from build123d import *

# Parameters (mm, degrees)
SKETCH_1_R          = 2.25
SKETCH_1_R_2        = 6
SKETCH_1_R_3        = 7.25
EXTRUDE_1_DEPTH     = 15
SKETCH_2_R          = 4.25
CUT_EXTRUDE_2_DEPTH = 8
SKETCH_3_R          = 3.4
CUT_EXTRUDE_3_DEPTH = 1188.655030604
SKETCH_4_R          = 5
CUT_EXTRUDE_4_DEPTH = 15


with BuildPart() as part:
    # 草图1 → 拉伸1 (new body)
    with BuildSketch(Plane.XY):
        with BuildLine():
            Line((1164.940753882, 1110.911631895), (1146.940753882, 1110.911631895))
            ThreePointArc((1146.940753882, 1110.911631895), (1143.405219976, 1109.4471658), (1141.940753882, 1105.911631895))
            Line((1141.940753882, 1105.911631895), (1141.940753882, 1045.911631895))
            Line((1141.940753882, 1045.911631895), (1145.440753882, 1045.911631895))
            Line((1145.440753882, 1045.911631895), (1145.440753882, 1020.911631895))
            ThreePointArc((1145.440753882, 1020.911631895), (1146.905219976, 1017.376097989), (1150.440753882, 1015.911631895))
            Line((1150.440753882, 1015.911631895), (1161.440753882, 1015.911631895))
            ThreePointArc((1161.440753882, 1015.911631895), (1164.976287788, 1017.376097989), (1166.440753882, 1020.911631895))
            Line((1166.440753882, 1020.911631895), (1166.440753882, 1045.911631895))
            Line((1166.440753882, 1045.911631895), (1185.940753882, 1045.911631895))
            Line((1185.940753882, 1045.911631895), (1185.940753882, 1060.411631895))
            Line((1185.940753882, 1060.411631895), (1165.827613848, 1060.411631895))
            ThreePointArc((1165.827613848, 1060.411631895), (1165.271903508, 1058.315850107), (1164.277525065, 1056.389110167))
            ThreePointArc((1164.277525065, 1056.389110167), (1164.426035256, 1053.42635052), (1161.46327561, 1053.574860711))
            ThreePointArc((1161.46327561, 1053.574860711), (1155.940753882, 1051.911631895), (1150.418232154, 1053.574860711))
            ThreePointArc((1150.418232154, 1053.574860711), (1147.455472508, 1053.42635052), (1147.603982698, 1056.389110167))
            ThreePointArc((1147.603982698, 1056.389110167), (1145.940753882, 1061.911631895), (1147.603982698, 1067.434153622))
            ThreePointArc((1147.603982698, 1067.434153622), (1147.455472508, 1070.396913269), (1150.418232154, 1070.248403078))
            ThreePointArc((1150.418232154, 1070.248403078), (1155.940753882, 1071.911631895), (1161.46327561, 1070.248403078))
            ThreePointArc((1161.46327561, 1070.248403078), (1164.426035256, 1070.396913269), (1164.277525065, 1067.434153622))
            ThreePointArc((1164.277525065, 1067.434153622), (1165.271903508, 1065.507413682), (1165.827613848, 1063.411631895))
            Line((1165.827613848, 1063.411631895), (1185.940753882, 1063.411631895))
            Line((1185.940753882, 1063.411631895), (1185.940753882, 1077.911631895))
            Line((1185.940753882, 1077.911631895), (1169.940753882, 1077.911631895))
            Line((1169.940753882, 1077.911631895), (1169.940753882, 1105.911631895))
            ThreePointArc((1169.940753882, 1105.911631895), (1168.476287788, 1109.4471658), (1164.940753882, 1110.911631895))
        make_face()
        with Locations((1162.940753882, 1104.911631895)):
            Circle(SKETCH_1_R, mode=Mode.SUBTRACT)
        with Locations((1155.940753882, 1097.911631895)):
            Circle(SKETCH_1_R_2, mode=Mode.SUBTRACT)
        with Locations((1148.940753882, 1104.911631895)):
            Circle(SKETCH_1_R, mode=Mode.SUBTRACT)
        with Locations((1148.940753882, 1090.911631895)):
            Circle(SKETCH_1_R, mode=Mode.SUBTRACT)
        with Locations((1162.940753882, 1090.911631895)):
            Circle(SKETCH_1_R, mode=Mode.SUBTRACT)
        with Locations((1155.940753882, 1026.411631895)):
            Circle(SKETCH_1_R_3, mode=Mode.SUBTRACT)
    extrude(amount=EXTRUDE_1_DEPTH)

    # 草图2 → 拉伸2 (cut)
    with BuildSketch(Plane(origin=(0, 0, 0), x_dir=(-1, 0, 0), z_dir=(0, 0, -1))):
        with Locations((-1148.940753882, 1090.911631895)):
            Circle(SKETCH_2_R)
        with Locations((-1162.940753882, 1090.911631895)):
            Circle(SKETCH_2_R)
        with Locations((-1148.940753882, 1104.911631895)):
            Circle(SKETCH_2_R)
        with Locations((-1162.940753882, 1104.911631895)):
            Circle(SKETCH_2_R)
    extrude(amount=-CUT_EXTRUDE_2_DEPTH, mode=Mode.SUBTRACT)

    # 草图3 → 拉伸3 (cut, through all)
    with BuildSketch(Plane(origin=(0, 1077.911631895, 0), x_dir=(1, 0, 0), z_dir=(0, 1, 0))):
        with Locations(Location((1177.940753882, -7.5, 0), (0, 0, 270))):
            Circle(SKETCH_3_R)
    extrude(amount=-CUT_EXTRUDE_3_DEPTH, mode=Mode.SUBTRACT)

    # 草图4 → 拉伸4 (cut)
    with BuildSketch(Plane(origin=(0, 1077.911631895, 0), x_dir=(1, 0, 0), z_dir=(0, 1, 0))):
        with Locations(Location((1177.940753882, -7.5, 0), (0, 0, 270))):
            Circle(SKETCH_4_R)
    extrude(amount=-CUT_EXTRUDE_4_DEPTH, mode=Mode.SUBTRACT)


solid = part.part
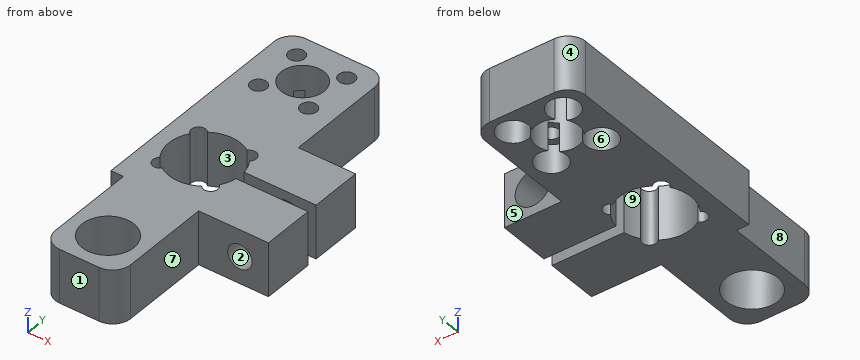
Work out the finished part from the listing and answer in its coordinate system (mm). Face numbers are marked on the shaded views. A direction names the side the tool comes from. Coordinates: 2 decimals unless noted, no trailing zeros. Write each loop counter-clockwise with the first axis right and the second up, starting at its lowest first coordinate (ties: lowest second). Pieces come first, ordered by that corner, then holes. Notation, with made-up numbers: M 81.5,59.5 L 87.5,59.5 A14 ccw 87.5,77.5 Z; hole C 32.25,-7 d6. An arc over 180 degrees is marked long. Write item = value, one per line.
1. The part is cut by section A-A (x = 1156). Determine the outline of the cut face in (y, z), then the cut area to 3 significant figures.
Solution:
outline = M 1015.91,0 L 1019.16,0 L 1019.16,15 L 1015.91,15 Z; M 1033.66,0 L 1051.91,0 L 1051.91,15 L 1033.66,15 Z; M 1071.91,0 L 1091.91,0 L 1091.91,15 L 1071.91,15 Z; M 1103.91,0 L 1110.91,0 L 1110.91,15 L 1103.91,15 Z
area = 728 mm2
2. The part is cut by section B-B (z = 6.75). State how many separate pieces and enclosed holes the cut face has, then the cut area to 3 significant figures.
Solution:
separate_pieces = 3
enclosed_holes = 2
area = 1,800 mm2
3. Straight lines are drawn through the part: line 1 (Y direction, x = 1155.5, z = 7.5); line 2 (Y direction, x = 1157, z = 8.5); line 3 (X direction, y = 1089.5, z = 7.25). For each, find the intervals that lie inside material, in ascending order. Write a range as from..to.
Solution:
line_1 = 1015.91..1019.18, 1033.65..1051.92, 1071.9..1091.93, 1103.9..1110.91
line_2 = 1015.91..1019.24, 1033.58..1051.97, 1071.86..1092.01, 1103.82..1110.91
line_3 = 1141.94..1144.93, 1152.95..1158.93, 1166.95..1169.94
4. The part is cut by section C-C (y = 1038). Determine the outline of the cut face in (x, z), then the cut area to 3 significant figures.
Solution:
outline = M 1145.44,0 L 1166.44,0 L 1166.44,15 L 1145.44,15 Z
area = 315 mm2
5. Flat-ended cylindrical pins translate along their axes: pin 1 (7 mm diameter, centred on x = 1162.94, y = 1104.91, fed in from -Z); pin 2 (4 mm diameter, centred on x = 1143, z = 7.5, fed in from -Y); pin 3 (4.5 mm diameter, centred on y = 1034, z = 10.5, fed in from -X). Find the tip coordinate at first contact, or state that the pin passes through.
Solution:
pin_1 = 8
pin_2 = 1045.91
pin_3 = 1145.44
6. For the marked faces 5, 6, 7, 8 and 9, determine the directions among +Z, -Z, +X, -X, +Y, -Y from which every point of the face is accessible in a straight line to the end or side of a thin tool.
Solution:
face_5 = +Z, -Z, +X, +Y
face_6 = -Z
face_7 = +Z, -Z, +X, -Y
face_8 = +Z, -Z, -X, -Y
face_9 = +Z, -Z
7. Determine the mould class of the marked faces 1, 2, 3 and 4 for opening direction Y: released by +Y, released by -Y, zero draft, split by the parting line, or undercut.
Solution:
face_1 = released by -Y
face_2 = zero draft
face_3 = undercut
face_4 = released by +Y
